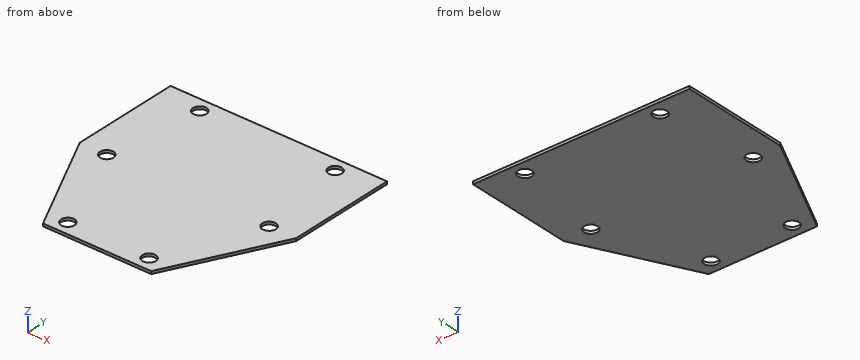
```python
from build123d import *

# Parameters (mm, degrees)
SKETCH1_R           = 2.5
BOSS_EXTRUDE1_DEPTH = 0.5


with BuildPart() as part:
    # Sketch1 → Boss-Extrude1 (new, symmetric)
    # profile 1 of 2: a face of its own
    with BuildSketch(Plane.XY):
        Polygon((0, 40), (0, -40), (20, -40), (40, 0), (40, 40), align=None)
        with Locations((15, -35)):
            Circle(SKETCH1_R, mode=Mode.SUBTRACT)
        with Locations((30, 0)):
            Circle(SKETCH1_R, mode=Mode.SUBTRACT)
        with Locations((25, 35)):
            Circle(SKETCH1_R, mode=Mode.SUBTRACT)
    # profile 2 of 2: a face of its own
    with BuildSketch(Plane.XY):
        Polygon((-20, -40), (0, -40), (0, 40), (-40, 40), (-40, 0), align=None)
        with Locations((-15, -35)):
            Circle(SKETCH1_R, mode=Mode.SUBTRACT)
        with Locations((-30, 0)):
            Circle(SKETCH1_R, mode=Mode.SUBTRACT)
        with Locations((-25, 35)):
            Circle(SKETCH1_R, mode=Mode.SUBTRACT)
    extrude(amount=BOSS_EXTRUDE1_DEPTH, both=True)


solid = part.part
```
Build history of the part. All positions in model axes, mm. Give positions to 0.01 mm unless a question says otherwise; leave off trailing zeros. Loops run counter-clockwise (first coordinate to the right, second up) from the corner with the lowest first, then second, coordinate; pieces in that order, holes last.
1) Band-saw the part on C-C on z = 0.3. List the corners of the cut face in (x, y).
Values follow:
outline: (-40, 0) - (-20, -40) - (20, -40) - (40, 0) - (40, 40) - (-40, 40) - close; hole circle Ø5 at (-30, 0); hole circle Ø5 at (-25, 35); hole circle Ø5 at (-15, -35); hole circle Ø5 at (15, -35); hole circle Ø5 at (25, 35); hole circle Ø5 at (30, 0)
2) Band-saw the part on B-B on y = 35. List the corners of the cut face in (x, z).
Values follow:
outline: (-40, -0.5) - (-27.5, -0.5) - (-27.5, 0.5) - (-40, 0.5) - close; (-22.5, -0.5) - (22.5, -0.5) - (22.5, 0.5) - (-22.5, 0.5) - close; (27.5, -0.5) - (40, -0.5) - (40, 0.5) - (27.5, 0.5) - close
3) Band-saw the part on D-D on x = -25. List the corners of the cut face in (y, z), then the cut area to 3 significant figures.
Values follow:
outline: (-30, -0.5) - (32.5, -0.5) - (32.5, 0.5) - (-30, 0.5) - close; (37.5, -0.5) - (40, -0.5) - (40, 0.5) - (37.5, 0.5) - close
area: 65.0 mm2
4) Band-saw the part on A-A on x = 30. List the corners of the cut face in (y, z).
Values follow:
outline: (-20, -0.5) - (-2.5, -0.5) - (-2.5, 0.5) - (-20, 0.5) - close; (2.5, -0.5) - (40, -0.5) - (40, 0.5) - (2.5, 0.5) - close
5) Drop a flat-ended pin along its axis: P1, Ø4.5, axis at x = -25, y = 35, coming from the +Z side. Give the stop position or say it passes through.
Values follow:
P1: passes through
6) Probe line 1 along Y through (x, z) = (30, 0.2); line 2 along Y through (x, z) = (-15, -0.3); line 3 along Y through (x, z) = (34, 0.1). List the from-to ranges inside material, lowest first.
Values follow:
line 1: y = -20 to -2.5, 2.5 to 40
line 2: y = -40 to -37.5, -32.5 to 40
line 3: y = -12 to 40
